Input: part model. Units: mm. Frame: model coordinates. Face numbers are marked on the shaded views. Give positions to 0.01 mm unless a question says otherwise; leave off trailing zeros. Write each loop counter-clockwise with the first axis right and the second up, starting at its lowest first coordinate (ties: lowest second). Pieces come first, ordered by that corner, then holes. Notation, with made-up numbers: (76.25, 70) - (130.25, 70) arc R24 cw to (130.25, 96) - close; hole circle Ø2 at (-27, 17.25). An arc over 180 degrees is marked (long way). Use a Markdown table: item, result. Add a question column.
1. Section query C-C, the plane z = -0.8. Return loops of the section in (x, y), plus the area to 3 significant figures.
2. Material intervals for probe 1 along Y at (x, z) = (-25.35, -0.6); probe 2 along Y at (x, z) = (-64.85, 1.05); probe 3 along X at (y, z) = (-20.75, -0.4), sorted ascending.
3. Section query A-A, the plane x = -25.35. Return loops of the section in (y, z).
4. Section query D-D, the plane y = -20.5. Return loops of the section in (x, z).
5. Mould query, pull axis Y, two halves, no side actions, for the marked faces 1, 2 and 3. Classes: released by +Y, released by -Y, zero draft, split by the parting line, or undercut.
6. Section query B-B, the plane y = -4.75. Return loops of the section in (x, z), plus the area to 3 significant figures.
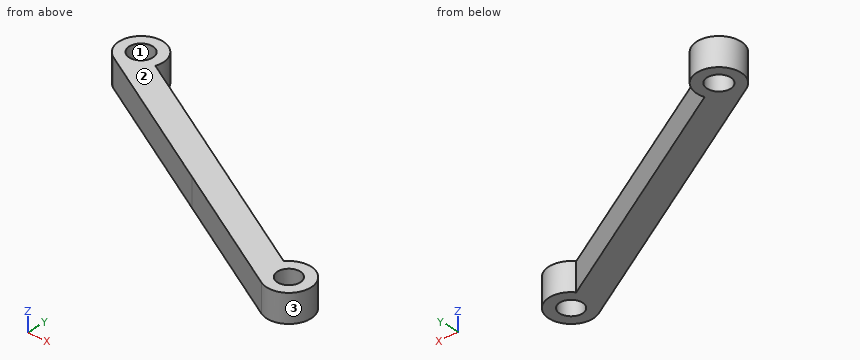
Autodesk Inventor part; units mm, degrees
ref_plane "YZ Plane" through (0, 0, 0) normal (1, 0, 0) x (0, 1, 0)
ref_plane "XZ Plane" through (0, 0, 0) normal (0, 1, 0) x (-1, 0, 0)
ref_plane "XY Plane" through (0, 0, 0) normal (0, 0, 1) x (1, 0, 0)
sketch "Sketch1" plane through (0, 0, 0) normal (0, 0, 1) x (1, 0, 0)
  circle A0 centre (-25.35, -26.8891) radius 1.55
  circle A1 centre (-25.35, -26.8891) radius 3
  circle A2 centre (-64.85, -5.4402) radius 1.6
  circle A3 centre (-64.85, -5.4402) radius 3
  line L0 (-26.7816, -29.5255) -> (-66.2816, -8.0766) construction
  line L1 (-23.9184, -24.2527) -> (-63.4184, -2.8038) construction
  line L2 (-26.7816, -29.5255) -> (-45.35, -19.4427)
  line L3 (-62.0119, -6.4124) -> (-62.0119, -6.4124)
  line L4 (-32.35, -16.7754) -> (-65.35, -16.7754)
  line L5 (-32.35, -5.7754) -> (-57.816, -5.7754)
  line L6 (-32.35, -5.7754) -> (-32.35, -16.7754) construction
  line L7 (-32.35, -11.2754) -> (-52.35, -11.2754) construction
  line L8 (-63.35, -10.6613) -> (-63.35, -16.3989) construction
  line L9 (-45.35, -19.4427) -> (-66.2816, -8.0766)
  line L10 (-62.0119, -6.4124) -> (-27.7109, -25.0381)
  point P0 (0, 0)
  point P1 (-47.8172, -11.2754)
  dimension "d0" = 6
  dimension "d1" = 6
  dimension "d10" = 20
  dimension "d11" = 20
  dimension "d19" = 3.5
extrude "Extrusion1" add sketch "Sketch1" along normal mid plane 3.8
properties part number "palanca base_proxima" material "PPS Plastic"
Result sheet:
| question | item | result |
|---|---|---|
| 1 | outline | (-66.28, -8.08) - (-45.35, -19.44) - (-26.78, -29.53) arc R3 ccw (long way) to (-27.71, -25.04) - (-62.01, -6.41) arc R3 ccw (long way) to start; hole circle Ø3.2 at (-64.85, -5.44); hole circle Ø3.1 at (-25.35, -26.89) |
| 1 | area | 181 mm² |
| 2 | probe 1 | y = -29.89 to -28.44, -25.34 to -23.89 |
| 2 | probe 2 | y = -8.85 to -7.04, -3.84 to -2.44 |
| 2 | probe 3 | x = -42.94 to -35.61 |
| 3 | outline | (-29.89, -1.9) - (-28.44, -1.9) - (-28.44, 1.9) - (-29.89, 1.9) - close; (-25.34, -1.9) - (-23.89, -1.9) - (-23.89, 1.9) - (-25.34, 1.9) - close |
| 4 | outline | (-43.4, -1.9) - (-36.07, -1.9) - (-36.07, 1.9) - (-43.4, 1.9) - close |
| 5 | face 1 | undercut |
| 5 | face 2 | zero draft |
| 5 | face 3 | split by the parting line |
| 6 | outline | (-67.77, -1.9) - (-66.29, -1.9) - (-66.29, 1.9) - (-67.77, 1.9) - close; (-63.41, -1.9) - (-61.93, -1.9) - (-61.93, 1.9) - (-63.41, 1.9) - close |
| 6 | area | 11.2 mm² |
